The listing builds one solid part. Answer for the finished solid, in the listing's coordinates (mm). A direction names the side the tool comes from. Round coordinates to 2 decimals unless told otherwise and drop trailing zeros. Write item = value, one per line.
from build123d import *

# Parameters (mm, degrees)
BOSS_EXTRUDE1_DEPTH = 4
SKETCH3_R           = 1.5
CUT_EXTRUDE1_DEPTH  = 10
SKETCH4_R           = 1.5
CUT_EXTRUDE2_DEPTH  = 137.530216436


with BuildPart() as part:
    # Sketch1 → Boss-Extrude1 (new body)
    with BuildSketch(Plane.XY):
        with BuildLine():
            Line((-96.5, -48), (-73.5, -48))
            Line((-73.5, -48), (-73.5, -23.206895527))
            ThreePointArc((-73.5, -23.206895527), (-82.3, 0), (-73.5, 23.206895527))
            Line((-73.5, 23.206895527), (-73.5, 27))
            Line((-73.5, 27), (-35.485281374, 27))
            Line((-35.485281374, 27), (-27, 35.485281374))
            Line((-27, 35.485281374), (-27, 73.5))
            Line((-27, 73.5), (-23.206895527, 73.5))
            ThreePointArc((-23.206895527, 73.5), (0, 82.3), (23.206895527, 73.5))
            Line((23.206895527, 73.5), (48, 73.5))
            Line((48, 73.5), (48, 96.5))
            Line((48, 96.5), (-52, 96.5))
            Line((-52, 96.5), (-96.5, 52))
            Line((-96.5, 52), (-96.5, -48))
        make_face()
    extrude(amount=BOSS_EXTRUDE1_DEPTH)

    # Sketch3 → Cut-Extrude1 (cut)
    with BuildSketch(Plane.XY.offset(4)):
        with Locations((30.5, 78.72592343)):
            Circle(SKETCH3_R)
        with Locations((30.5, 88.72592343)):
            Circle(SKETCH3_R)
        with Locations((42.5, 88.72592343)):
            Circle(SKETCH3_R)
        with Locations((42.5, 78.72592343)):
            Circle(SKETCH3_R)
        with Locations((-42.5, 78.72592343)):
            Circle(SKETCH3_R)
        with Locations((-42.5, 88.72592343)):
            Circle(SKETCH3_R)
        with Locations((-30.5, 88.72592343)):
            Circle(SKETCH3_R)
        with Locations((-30.5, 78.72592343)):
            Circle(SKETCH3_R)
        with Locations((-88.72592343, 30.5)):
            Circle(SKETCH3_R)
        with Locations((-88.72592343, 42.5)):
            Circle(SKETCH3_R)
        with Locations((-78.72592343, 42.5)):
            Circle(SKETCH3_R)
        with Locations((-78.72592343, 30.5)):
            Circle(SKETCH3_R)
        with Locations((-88.72592343, -42.5)):
            Circle(SKETCH3_R)
        with Locations((-88.72592343, -30.5)):
            Circle(SKETCH3_R)
        with Locations((-78.72592343, -30.5)):
            Circle(SKETCH3_R)
        with Locations((-78.72592343, -42.5)):
            Circle(SKETCH3_R)
    extrude(amount=-CUT_EXTRUDE1_DEPTH, mode=Mode.SUBTRACT)

    # Sketch4 → Cut-Extrude2 (cut, through all)
    with BuildSketch(Plane.XY.offset(4)):
        with Locations((-88, 0)):
            Circle(SKETCH4_R)
        with Locations((-63.639610307, 63.639610307)):
            Circle(SKETCH4_R)
        with Locations((0, 88)):
            Circle(SKETCH4_R)
        with Locations((-80.960118382, 53.639610307)):
            Circle(SKETCH4_R)
        with Locations((-53.639610307, 80.960118382)):
            Circle(SKETCH4_R)
        with Locations((19.318516526, 82.823619098)):
            Circle(SKETCH4_R)
        with Locations((-19.318516526, 82.823619098)):
            Circle(SKETCH4_R)
        with Locations((-82.823619098, 19.318516526)):
            Circle(SKETCH4_R)
        with Locations((-82.823619098, -19.318516526)):
            Circle(SKETCH4_R)
        with Locations((-40.658639918, 65.40737726)):
            Circle(SKETCH4_R)
        with Locations((-65.40737726, 40.658639918)):
            Circle(SKETCH4_R)
        with Locations((-49.497474683, 35.355339059)):
            Circle(SKETCH4_R)
        with Locations((-35.355339059, 49.497474683)):
            Circle(SKETCH4_R)
    extrude(amount=-CUT_EXTRUDE2_DEPTH, mode=Mode.SUBTRACT)


solid = part.part
Q1. Determine the mould class of faces 1 (the face through (-73.5, -36, 2)), 2 (the face through (-0.36, 82.3, 1.97)), 3 (the face through (35, 73.5, 2)), 4 (the face through (-96.5, 3, 2)) for opening direction X: released by +X, released by -X, zero draft, split by the parting line, or undercut.
Model answer:
face_1 = released by +X
face_2 = undercut
face_3 = zero draft
face_4 = released by -X
Q2. For faces 5 (the face through (-25, 73.5, 2)), 6 (the face through (-1, 96.5, 2)), determine the directions among +Z, -Z, +X, -X, +Y, -Y from which every point of the face is accessible in a straight line to the end or side of a thin tool.
Model answer:
face_5 = +Z, -Z, +X, -Y
face_6 = +Z, -Z, +X, -X, +Y
Q3. Section A-A on z = 1 is taken. Count the separate pieces of the cut face and the enclosed holes in it, then the cut area to 3 significant figures.
Model answer:
separate_pieces = 1
enclosed_holes = 29
area = 6,490 mm^2
Q4. Find the intervals of material crossed by line 1 (Y direction, x = 42.5, z = 2.9); line 2 (Y direction, x = 41.5, z = 1.45); line 3 (X direction, y = 42, z = 1), in increasing order. Write a range as from..to.
Model answer:
line_1 = 73.5..77.23, 80.23..87.23, 90.23..96.5
line_2 = 73.5..77.61, 79.84..87.61, 89.84..96.5
line_3 = -96.5..-90.14, -87.31..-80.14, -77.31..-66.08, -64.74..-27
Q5. Flat-ended cylindrical pins translate along their axes: P1, Ø2, axis at y = -40, z = 1.5, coming from the +X side; P2, Ø1.2, axis at x = -45.5, z = 1.5, coming from the -Y side. Find the tip coordinate at first contact, or state that the pin passes through.
Model answer:
P1 = -73.5
P2 = 27
